The drawing under review shows one solid part. Ordinate dimensions are in mm from its lowest x, y, z. Coordinates: 2 decimals unless noted, no trailing zeros. Write each loop counter-clockwise with the first axis right and the second up, starting at its lowest first coordinate (ties: lowest second). Pieces come first, ordered by that corner, then holes.
Q1. For probe 1 along X at (y, z) = (1.7, 10.5) (1 decimal); probe 2 along X at (y, z) = (0.9, 8) (1 decimal); probe 3 along Z at (x, y) = (3.5, 1.55) (1 decimal), list the stretches that pass through material, from the lowest coordinate up.
Q2. Take a section at A-A (x = 8). Give the boundary of the cut face in (y, z) (1 decimal), and give its area (3 significant figures).
Q3. Take a section at D-D (z = 11.25). Give the boundary of the cut face in (x, y), and give its area (3 significant figures).
Q4. Take a section at C-C (y = 2). Give the boundary of the cut face in (x, z) (1 decimal).
Q5. Take a section at B-B (z = 5.5). Give the boundary of the cut face in (x, y) (1 decimal).
Q6. Mouldability with a two-part tool opening along Z and no side actions: class the marked faces 1, 2, 3 and 4 as pulls with the +Z half, pulls with the -Z half, needs draft (parallel to the pull), parting line crosses it, or undercut.
Q7. Insertion check: pin 1 (1.5 mm diameter, centred on x = 9, y = 2.5, fed in from -Z); pin 2 (1 mm diameter, centred on x = 9.5, y = 2, fed in from -Z); pin 3 (1 mm diameter, centred on x = 10.5, y = 2.5, fed in from -Z); pin 4 (5 mm diameter, centred on x = 6.06, z = 6.85, fed in from +Y). Each pin has a flat end and moves straight along its axis. Give the tip position at first contact, or say it passes through.
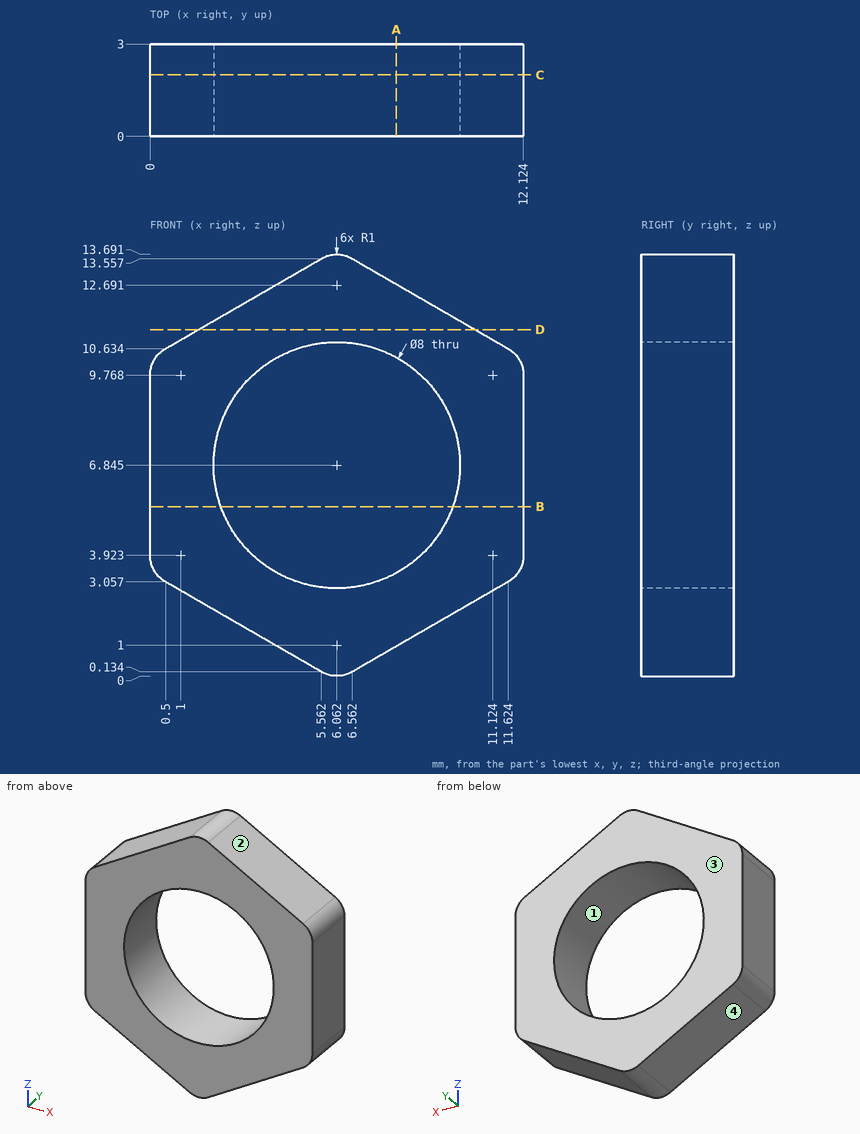
Response:
1. probe 1: x = 0.3 to 4.4, 7.7 to 11.8
1. probe 2: x = 0 to 2.2, 9.9 to 12.1
1. probe 3: z = 1.3 to 3.8, 9.9 to 12.4
2. outline: (0, 1) - (3, 1) - (3, 3.3) - (0, 3.3) - close; (0, 10.3) - (3, 10.3) - (3, 12.7) - (0, 12.7) - close
2. area: 14.3 mm2
3. outline: (1.57, 0) - (10.56, 0) - (10.56, 3) - (1.57, 3) - close
3. area: 27.0 mm2
4. outline: (0, 3.9) arc R1 ccw to (0.5, 3.1) - (5.6, 0.1) arc R1 ccw to (6.6, 0.1) - (11.6, 3.1) arc R1 ccw to (12.1, 3.9) - (12.1, 9.8) arc R1 ccw to (11.6, 10.6) - (6.6, 13.6) arc R1 ccw to (5.6, 13.6) - (0.5, 10.6) arc R1 ccw to (0, 9.8) - close; hole circle Ø8 at (6.1, 6.8)
5. outline: (0, 0) - (2.3, 0) - (2.3, 3) - (0, 3) - close; (9.8, 0) - (12.1, 0) - (12.1, 3) - (9.8, 3) - close
6. face 1: undercut
6. face 2: pulls with the +Z half
6. face 3: needs draft
6. face 4: pulls with the -Z half
7. pin 1: stops at z = 1.11
7. pin 2: stops at z = 1.54
7. pin 3: stops at z = 2.12
7. pin 4: passes through
